Geometry check sheet. Reference: the model listing, model coordinates, mm. A direction names the side the tool comes from. Round coordinates to 2 decimals unless told otherwise and drop trailing zeros. Order: outer loops, then holes, each group sorted by start corner. A loop starts at its lowest first (then second) coordinate and runs counter-clockwise, first axis right, second up.
(1) Material ranges on line 1 along X through (y, z) = (0, 33.25); line 2 along Z through (x, y) = (8.75, -3.5), recorded low to high.
(2) Sectioned sample at B-B (z = -46). Record the boundary of the cut face in (x, y), plus the area to 3 significant figures.
(3) Sectioned sample at A-A (z = 18). Record the boundary of the cut face in (x, y), plus the area to 3 significant figures.
(4) Set-up check for faces 4 (the face through (-3.584, -2.285, -40.422)), 5 (the face through (8.5, 0, 0)), 6 (the face through (-8.5, 0, 0)), 7 (the face through (0.72, 0.16, 25.89)): record each of +Z, -Z, +X, -X, +Y, -Y from which the full face is reachable in a straight line by a thin tool's end or side.
(5) Release check for a two-part mould opening along Y. For faces 1 (the face through (-8, -6, 1)), 2 (the face through (2, -4, 52.5)), 3 (the face through (-3.584, -2.285, 40.422)) record: +Y half, -Y half, draft (parallel to the pull), parting line (faces both ways), or undercut.
(6) Go/stop test with flat-tipped pins: pin 1 (12 mm diameter, centred on x = -7.5, z = -38, fed in from +Y); pin 2 (5 mm diameter, centred on x = -3.5, z = -6, fed in from -Y); pin 3 (6 mm diameter, centred on y = -6.5, z = -5.5, fed in from -X). Record where each tip stops, or that it passes through.
(7) Sectioned sample at C-C (y = -7). Record the boundary of the cut face in (x, z), plus the area to 3 significant figures.
from build123d import *

# Parameters (mm, degrees)
SKETCH_1_R          = 10
EXTRUDE_1_DEPTH     = 52.5
SKETCH_2_W          = 3
SKETCH_2_H          = 20
CUT_EXTRUDE_1_DEPTH = 30


with BuildPart() as part:
    # 草图1 → 凸台-拉伸1 (new body, symmetric)
    with BuildSketch(Plane.XY):
        Circle(SKETCH_1_R)
    extrude(amount=EXTRUDE_1_DEPTH, both=True)

    # 草图2 → 切除-拉伸1 (cut, symmetric)
    with BuildSketch(Plane(origin=(0, 0, 0), x_dir=(1, 0, 0), z_dir=(0, 1, 0))):
        with Locations((-10, 0)):
            Rectangle(SKETCH_2_W, SKETCH_2_H)
        with Locations((10, 0)):
            Rectangle(SKETCH_2_W, SKETCH_2_H)
    extrude(amount=CUT_EXTRUDE_1_DEPTH, both=True, mode=Mode.SUBTRACT)

    # 草图4 → M10 螺纹孔1 (revolve, cut)
    with BuildSketch(Plane(origin=(0, 0, 52.5), x_dir=(0, -1, 0), z_dir=(1, 0, 0))):
        Polygon((0, 0), (0, 27.053657631), (4.25, 24.5), (4.25, 0), align=None)
    hole_wizard_m10_1 = revolve(axis=Axis((0, 0, 58.85), (0, 0, -1)), mode=Mode.SUBTRACT)

    # 镜向1: M10 螺纹孔1 across plane
    add(hole_wizard_m10_1.mirror(Plane.XY), mode=Mode.SUBTRACT)


solid = part.part
Answer below:
1. line 1: x = -10 to -4.25, 4.25 to 10
1. line 2: z = -52.5 to -10, 10 to 52.5
2. outline: circle Ø20 at (0, 0); hole circle Ø8.5 at (0, 0)
2. area: 257 mm2
3. outline: circle Ø20 at (0, 0)
3. area: 314 mm2
4. face 4: -Z
4. face 5: +X, +Y, -Y
4. face 6: -X, +Y, -Y
4. face 7: +Z
5. face 1: parting line
5. face 2: draft
5. face 3: undercut
6. pin 1: stops at y = 9.89
6. pin 2: stops at y = -9.95
6. pin 3: stops at x = -8.5
7. outline: (-7.14, -52.5) - (7.14, -52.5) - (7.14, 52.5) - (-7.14, 52.5) - close
7. area: 1,500 mm2
